Part print with two shaded views. Sizes in mm from the minimum x, y, z corner. Round coordinates to 2 decimals unless told otherwise and drop trailing zeros. Order: outer loops, then holes, each group sorted by start corner. A loop starts at its lowest first (then second) coordinate and runs counter-clockwise, first axis right, second up. Notation, with made-up numbers: (84.5, 29) - (120.5, 29) arc R11 ccw to (120.5, 35) - close; hole circle Ø6 at (-5, 73). An arc over 180 degrees is marked (long way). Write item = value, one per line.
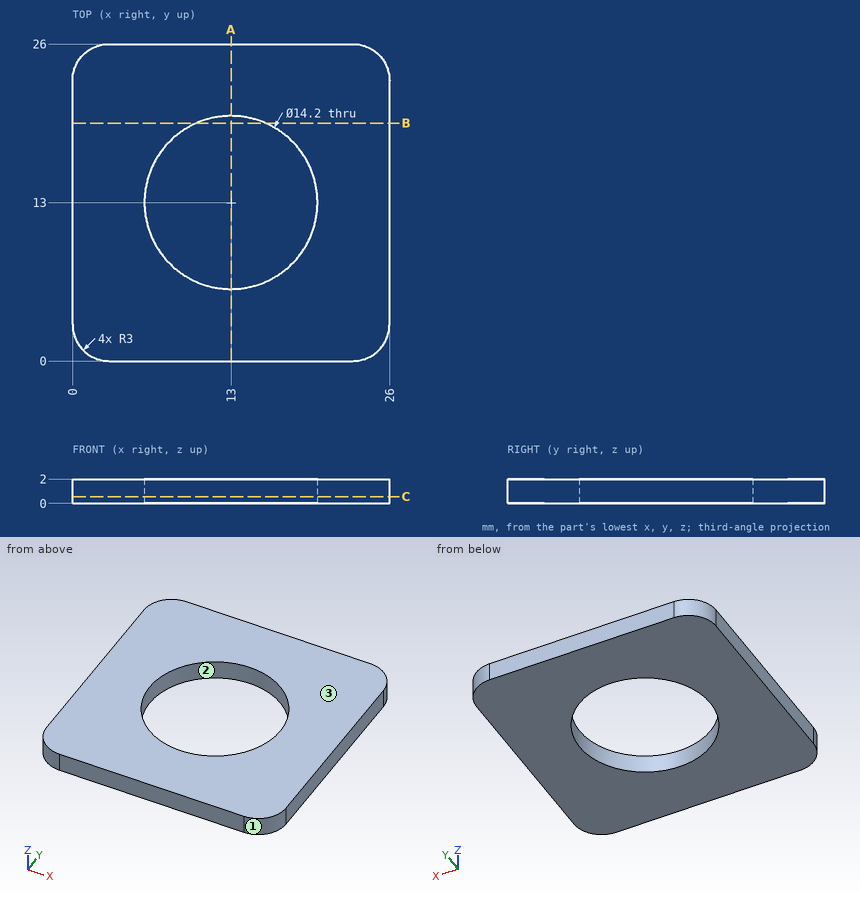
1) Cut at B-B (y = 19.5). Write the cut outline in (x, z), and give its area (3 significant figures).
Conclusion:
outline = (0, 0) - (10.14, 0) - (10.14, 2) - (0, 2) - close; (15.86, 0) - (26, 0) - (26, 2) - (15.86, 2) - close
area = 40.6 mm^2
2) Cut at C-C (z = 0.55). Write the cut outline in (x, y).
Conclusion:
outline = (0, 3) arc R3 ccw to (3, 0) - (23, 0) arc R3 ccw to (26, 3) - (26, 23) arc R3 ccw to (23, 26) - (3, 26) arc R3 ccw to (0, 23) - close; hole circle Ø14.2 at (13, 13)
3) Cut at A-A (x = 13). Write the cut outline in (y, z).
Conclusion:
outline = (0, 0) - (5.9, 0) - (5.9, 2) - (0, 2) - close; (20.1, 0) - (26, 0) - (26, 2) - (20.1, 2) - close
4) Wall check: line 1 along Y through (x, z) = (13, 1.35); line 2 along X through (y, z) = (13.75, 0.75); line 3 along X through (y, z) = (7.75, 0.55). Give the ranges that are in metal, low to high.
Conclusion:
line_1 = 0 to 5.9, 20.1 to 26
line_2 = 0 to 5.94, 20.06 to 26
line_3 = 0 to 8.22, 17.78 to 26
5) Mould opens along X. For the marked faces 1, 2 and 3 say: +X half, -X half, draft (parallel to the pull), parting line (faces both ways), or undercut.
Conclusion:
face_1 = +X half
face_2 = undercut
face_3 = draft
